Source: CAD feature listing. Evaluate the final solid. Frame: model axes, mm. A direction names the side the tool comes from. Give positions to 0.01 mm unless a question says otherwise; leave off trailing zeros. Order: outer loops, then holes, each group sorted by start corner. A loop starts at its lowest first (then second) coordinate and runs counter-clockwise, first axis right, second up. Notation, with made-up numbers: (65, 33) - (90, 33) arc R19 ccw to (90, 40) - close; hole circle Ø5 at (-2, 48). An arc over 180 degrees is marked (long way). Write each question's results on one line, items separated by ' | '. Start each with the question number.
Item 1: Section B-B on x = 31.75. Output: boundary loops of the cut face in (y, z) (3 decimals).
Item 2: Section C-C on z = -20.5. State how many separate pieces and enclosed holes the cut face has, and give its area (3 significant figures).
Item 3: Mould query, pull axis X, two halves, no side actions, for faces 1 (the flat face through (46, 2, 0)), 2 (the cylindrical face through (36.312, 1.61, -25.475)), 3 (the cylindrical face through (0.91, 1.57, -15.1)), 4 (the cylindrical face through (70.84, 1.61, -0.95)). Classes: released by +X, released by -X, zero draft, split by the parting line, or undercut.
Item 4: Contact query for flat-ended pins moving along their axis: pin 1 Ø11 at (x, z) = (31.75, -20.5) entering from -Y; pin 2 Ø10 at (x, z) = (8, -20.5) entering from -Y; pin 3 Ø1 at (y, z) = (1, -9) entering from -X. Output: stop coordinate, or through.
Item 5: Set-up query: faces 5 (the flat face through (11, 2, -14.15)), 6 (the flat face through (43, 0, -16)). Return all of +Z, -Z, +X, -X, +Y, -Y with unobstructed straight access to the full face (end or side cutting, diameter ignored); none if empty.
Item 6: Line query: line 1 along X through (y, z) = (0.8, -20.5); line 2 along Z through (x, y) = (8, 1.3); line 3 along X through (y, z) = (0.75, -22). Output: solid intervals per line, ascending.
```python
from build123d import *

# Parameters (mm, degrees)
SKETCH1_W             = 71.75
SKETCH1_H             = 32.5
BOSS_EXTRUDE1_DEPTH   = 3.175
M4X0_7_TAPPED_HOLE1_D = 3.3
SKETCH5_R             = 6.75
CUT_EXTRUDE1_DEPTH    = 79.831422193
SKETCH6_W             = 21.4
SKETCH6_H             = 14.15
CUT_EXTRUDE2_DEPTH    = 79.831422193
FILLET1_R             = 3.175


with BuildPart() as part:
    # Sketch1 → Boss-Extrude1 (new body)
    with BuildSketch(Plane(origin=(0, 0, 0), x_dir=(1, 0, 0), z_dir=(0, 1, 0))):
        with Locations((35.875, 16.25)):
            Rectangle(SKETCH1_W, SKETCH1_H)
    extrude(amount=BOSS_EXTRUDE1_DEPTH)

    # M4x0.7 Tapped Hole1 (through all)
    with Locations(Plane(origin=(0, 3.175, 0), x_dir=(1, 0, 0), z_dir=(0, 1, 0))):
        with Locations((7.9375, 20.5), (55.5625, 20.5), (55.5625, 5.26)):
            Hole(M4X0_7_TAPPED_HOLE1_D / 2)

    # Sketch5 → Cut-Extrude1 (cut, through all)
    with BuildSketch(Plane(origin=(0, 3.175, 0), x_dir=(1, 0, 0), z_dir=(0, 1, 0))):
        with Locations(Location((31.75, 20.5, 0), (0, 0, 270))):
            Circle(SKETCH5_R)
    extrude(amount=-CUT_EXTRUDE1_DEPTH, mode=Mode.SUBTRACT)

    # Sketch6 → Cut-Extrude2 (cut, through all)
    with BuildSketch(Plane(origin=(0, 3.175, 0), x_dir=(1, 0, 0), z_dir=(0, 1, 0))):
        with Locations((10.7, 7.075)):
            Rectangle(SKETCH6_W, SKETCH6_H)
    extrude(amount=-CUT_EXTRUDE2_DEPTH, mode=Mode.SUBTRACT)

    # Fillet1
    fillet1_edges = [part.edges().sort_by_distance(p)[0] for p in [
        (0, 1.5875, -14.15),
        (21.4, 1.5875, -14.15),
        (21.4, 1.5875, 0),
        (0, 1.5875, -32.5),
        (71.75, 1.5875, -32.5),
        (71.75, 1.5875, 0),
    ]]
    fillet(fillet1_edges, radius=FILLET1_R)


solid = part.part
```
Evaluation:
1) outline: (0, -32.5) - (3.175, -32.5) - (3.175, -27.25) - (0, -27.25) - close; (0, -13.75) - (3.175, -13.75) - (3.175, 0) - (0, 0) - close
2) separate pieces: 4 | enclosed holes: 0 | area: 164 mm^2
3) face 1: zero draft | face 2: undercut | face 3: released by -X | face 4: released by +X
4) pin 1: passes through | pin 2: stops at y = 0 | pin 3: stops at x = 21.4
5) face 5: +Z, -X, +Y, -Y | face 6: +Z, -Z, +X, -X, -Y
6) line 1: x = 0 to 6.29, 9.59 to 25, 38.5 to 53.91, 57.21 to 71.75 | line 2: z = -32.5 to -22.15, -18.85 to -14.15 | line 3: x = 0 to 7.25, 8.62 to 25.17, 38.33 to 54.88, 56.25 to 71.75
